Autodesk Inventor part; units mm, degrees
ref_plane "YZ Plane" through (0, 0, 0) normal (1, 0, 0) x (0, 1, 0)
ref_plane "XZ Plane" through (0, 0, 0) normal (0, 1, 0) x (-1, 0, 0)
ref_plane "XY Plane" through (0, 0, 0) normal (0, 0, 1) x (1, 0, 0)
sketch "Esboço1" plane through (0, 0, 0) normal (0, 0, 1) x (1, 0, 0)
  line L0 (0, 0) -> (64, 0)
  line L1 (64, 0) -> (64, 45)
  line L2 (64, 45) -> (0, 45)
  line L3 (0, 45) -> (0, 0)
  dimension "d0" = 64
  dimension "d1" = 45
extrude "Extrusão1" add sketch "Esboço1" against normal blind 32
sketch "Esboço2" plane through (0, 0, 0) normal (0, 0, 1) x (1, 0, 0)
  line L0 (0, 0) -> (0, 9)
  line L1 (0, 0) -> (0, 45)
  line L2 (0, 9) -> (24, 9)
  line L3 (24, 9) -> (24, 0)
  line L4 (24, 0) -> (40, 0)
  line L5 (64, 0) -> (0, 0)
  line L6 (40, 0) -> (40, 9)
  line L7 (40, 9) -> (64, 9)
  line L8 (64, 45) -> (64, 0)
  line L9 (0, 9) -> (0, 16)
  line L10 (64, 9) -> (64, 16)
  circle A0 centre (32, 29) radius 16
  line L11 (45.4187, 37.7142) -> (59.5201, 16)
  line L12 (18.5813, 37.7142) -> (4.4799, 16)
  line L13 (0, 16) -> (4.4799, 16)
  line L14 (59.5201, 16) -> (64, 16)
  line L15 (0, 16) -> (0, 45)
  line L16 (64, 45) -> (0, 45)
  line L17 (64, 45) -> (64, 16)
  point P0 (32, 45)
  dimension "d4" = 9
  dimension "d9" = 7
extrude "Extrusão2" cut sketch "Esboço2" against normal blind 22 contours L0 L2 L3 L5 | L1 L16 A0 L12 L13 | L6 L7 L8 L5 | L16 L8 L14 L11 A0
sketch "Esboço3" plane through (0, 0, 0) normal (0, 0, 1) x (1, 0, 0)
  line L0 (0, 0) -> (64, 0)
  line L1 (32, 0) -> (32, 29)
  point P0 (24, 0)
  point P1 (40, 0)
  dimension "d16" = 29
hole "Furo1" at (32, 29, 0) direction (0, 0, -1) diameter 12 depth 24
fillet "Arredondamento1" radius 3 2 edges at (4.4799, 16, -11) (59.5201, 16, -11)
sketch "Esboço5" plane through (0, 45, 0) normal (0, 1, 0) x (1, 0, 0)
  line L0 (64, 32) -> (0, 32)
  line L1 (0, 0) -> (0, 32)
  line L2 (0, 32) -> (0, 10)
  line L3 (0, 10) -> (32, 10)
  dimension "d30" = 22
hole "Furo2" at (32, 45, -10) direction (0, -1, 0) diameter 4.917 depth 11 tip angle 118 counterbore diameter 10.5 counterbore depth 4
sketch "Esboço6" plane through (0, 0, -32) normal (0, -1, 0) x (1, 0, 0)
  line L0 (45.4187, 32) -> (18.5813, 32)
  line L1 (32, 24) -> (32, 8)
  line L2 (38, 8) -> (26, 8)
  point P0 (0, 32)
  dimension "d40" = 16
hole "Furo3" at (32, 0, -8) at (32, 0, -24) direction (0, 1, 0) diameter 4.917 depth 12 tip angle 118
sketch "Sketch7" plane through (0, 0, -32) normal (0, -1, 0) x (1, 0, 0)
  line L0 (24, 32) -> (24, 10)
  line L1 (24, 10) -> (24, 0)
  line L2 (64, 0) -> (0, 0)
  line L3 (0, 0) -> (24, 0)
  line L4 (0, 10) -> (0, 0)
  line L5 (0, 0) -> (0, 10)
  line L6 (24, 10) -> (0, 10)
  line L7 (0, 10) -> (24, 10)
  line L8 (40, 32) -> (40, 10)
  line L9 (40, 10) -> (40, 0)
  line L10 (40, 0) -> (64, 0)
  line L11 (64, 10) -> (64, 0)
  line L12 (64, 0) -> (64, 10)
  line L13 (64, 10) -> (40, 10)
  line L14 (64, 10) -> (40, 10)
  point P0 (0, 32)
extrude "Extrusion3" cut sketch "Sketch7" against normal blind 9
properties part number "mordente_movel" material "Iron, Cast"
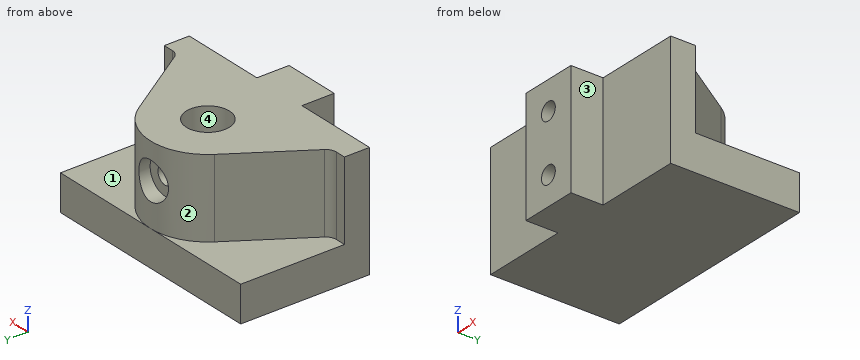
Part model, mm, in its own coordinate system. Face numbers are marked on the shaded views. A direction names the side the tool comes from. Round coordinates to 2 decimals unless told otherwise and drop trailing zeros. Loops run counter-clockwise (first coordinate to the right, second up) from the corner with the lowest first, then second, coordinate; pieces in that order, holes last. Notation, with made-up numbers: (72, 7) -> (111, 7) arc R24 ccw to (111, 34) -> close; hole circle Ø10 at (76, 59). An arc over 180 degrees is marked (long way). Use CSV: the item, a comma, the result in double quotes. Start each with the question number.
1) Which spindle directions (+Z, -Z, +X, -X, +Y, -Y) get a long thin tool onto all of the face, cutting with end or side? Do the marked faces 1, 2, 3 and 4. Say none if no direction does.
2) Cut at A-A, the plane y = 10. Write the cut outline in (x, z), plus the area to 3 significant figures.
3) Wall check: L1, parallel to Z at x = 32, y = 3; L2, parallel to Z at x = 32, y = 39.5; L3, parallel to X at y = 3, z = -8. Give the ranges that are in metal, low to high. Write a range as [from, to].
4) Cut at B-B, the plane x = 13. Write the cut outline in (y, z).
5) Cut at C-C, the plane x = 41. Write the cut outline in (y, z).
6) Drop flat-ended pins along their axis: P1, Ø4, axis at x = 32, z = -8, coming from the +Y side; P2, Ø10, axis at x = 14, z = -22, coming from the -Y side; P3, Ø2, axis at x = 52, y = 33, coming from the +Z side. Give the stop position or say it passes through.
Determined:
1,face 1,"+Z, +X, +Y"
1,face 2,"+Z, +Y"
1,face 3,"+Z, -Z, +X, -Y"
1,face 4,"+Z"
2,outline,"(0, -32) -> (64, -32) -> (64, 0) -> (0, 0) -> close; hole circle Ø4.92 at (32, -24); hole circle Ø4.92 at (32, -8)"
2,area,"2,010 mm2"
3,L1,"z = [-32, -26.46], [-21.54, -10.46], [-5.54, 0]"
3,L2,"z = [-32, -12.46], [-7.54, 0]"
3,L3,"x = [24, 29.54], [34.46, 40]"
4,outline,"(9, -32) -> (45, -32) -> (45, -22) -> (29.12, -22) -> (29.12, 0) -> (9, 0) -> close"
5,outline,"(9, -32) -> (45, -32) -> (45, -22) -> (42.23, -22) -> (42.23, 0) -> (9, 0) -> close"
6,P1,"stops at y = 41"
6,P2,"stops at y = 9"
6,P3,"stops at z = -22"
